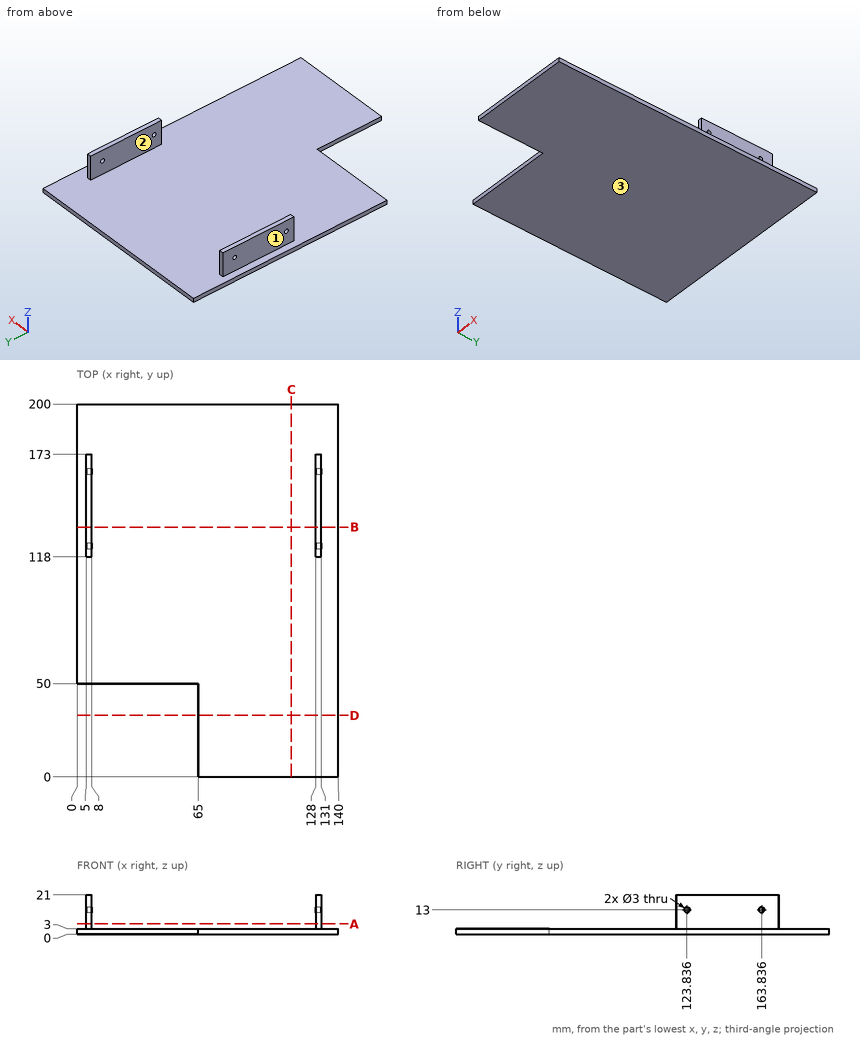
Print and shaded views of the part. All mm, measured from the part's lowest x, y and z. Coordinates: 2 decimals unless noted, no trailing zeros. Write each loop counter-clockwise with the first axis right and the second up, starting at its lowest first coordinate (ties: lowest second). Pieces come first, ordered by that corner, then holes.
(1) Cut at B-B, the plane y = 134. List the corners of the cut face in (x, z), and give its area (3 significant figures).
(2) Cut at A-A, the plane z = 5.5. List the corners of the cut face in (x, y), and give its area (3 significant figures).
(3) Cut at C-C, the plane x = 115. List the corners of the cut face in (y, z).
(4) Drill centre lines: probe 1 along Y at (x, z) = (130, 13) (1 decimal); probe 2 along X at (y, z) = (171, 14); probe 3 along Z at (x, y) = (73, 46). Where is each one in solid material? Low to high.
(5) Cut at D-D, the plane y = 33. List the corners of the cut face in (x, z).
(6) Two-plate mould, pull along X, no slides. Class the marked faces 1, 2 and 3: +X half, -X half, draft (parallel to the pull), parting line (faces both ways), or undercut.
(7) Flat gauge pins, fed straight in: pin 1 (10 mm diameter, centred on y = 85, z = 10.5, fed in from -X); pin 2 (3.5 mm diameter, centred on y = 123.84, z = 13, fed in from -X); pin 3 (2.5 mm diameter, centred on x = 45.5, z = 1.5, fed in from -Y); pin 4 (9 mm diameter, centred on y = 156.5, z = 13, fed in from +X). Where does each tip first touch, or does it go through?
Geometry says:
1. outline: (0, 0) - (140, 0) - (140, 3) - (131, 3) - (131, 21) - (128, 21) - (128, 3) - (8, 3) - (8, 21) - (5, 21) - (5, 3) - (0, 3) - close
1. area: 528 mm2
2. outline: (5, 118) - (8, 118) - (8, 173) - (5, 173) - close; (128, 118) - (131, 118) - (131, 173) - (128, 173) - close
2. area: 330 mm2
3. outline: (0, 0) - (200, 0) - (200, 3) - (0, 3) - close
4. probe 1: y = 118 to 122.3, 125.3 to 162.3, 165.3 to 173
4. probe 2: x = 5 to 8, 128 to 131
4. probe 3: z = 0 to 3
5. outline: (65, 0) - (140, 0) - (140, 3) - (65, 3) - close
6. face 1: -X half
6. face 2: undercut
6. face 3: draft
7. pin 1: passes through
7. pin 2: stops at x = 5
7. pin 3: stops at y = 50
7. pin 4: stops at x = 131
